CAD build for the part. Positions are in the model's coordinates, mm. A direction names the side the tool comes from. Give positions to 0.01 mm unless a question says otherwise; leave off trailing zeros. Loops run counter-clockwise (first coordinate to the right, second up) from the corner with the lowest first, then second, coordinate; pieces in that order, holes last.
Item 1: Drop flat-ended pins along their axis: P1, Ø1, axis at y = -1, z = 2, coming from the -X side; P2, Ø2, axis at y = -1.5, z = 1.5, coming from the -X side; P3, Ø1.5, axis at y = -0.5, z = 2, coming from the +X side. Give the stop position or say it passes through.
Item 2: Saw through at D-D on z = 0.25. Give the cut face in (x, y), plus the area to 3 significant figures.
Item 3: Saw through at C-C on x = 0. Give the cut face in (y, z), plus the area to 3 significant figures.
Item 4: Saw through at B-B on y = 0. Give the cut face in (x, z).
Item 5: Saw through at A-A on z = -2.25. Give the cut face in (x, y).
Item 6: Probe probe 1 along Y at (x, z) = (-1.2, 0.75); probe 2 along Y at (x, z) = (1.25, -0.25); probe 3 along Z at (x, y) = (0.6, -1.65). List the from-to ranges inside material, lowest first.
Item 7: Which spindle directions (+Z, -Z, +X, -X, +Y, -Y) get a long thin tool onto all of the face, cutting with end or side? Do faces 1 (the cylindrical face through (-1.5, 0.07, 2.28)), 2 (the flat face through (1.727, 0, 0.5)). Say none if no direction does.
from build123d import *

# Parameters (mm, degrees)
SKETCH1_R           = 2
BOSS_EXTRUDE1_DEPTH = 1
SKETCH2_R           = 1.5
BOSS_EXTRUDE2_DEPTH = 4
FILLET1_R           = 1.5
SKETCH3_W           = 0.5
SKETCH3_H           = 0.5
BOSS_EXTRUDE3_DEPTH = 4
FILLET2_R           = 0.2
FILLET3_R           = 0.1
FILLET4_R           = 0.1
CUT_EXTRUDE1_DEPTH  = 6


with BuildPart() as part:
    # Sketch1 → Boss-Extrude1 (new body)
    with BuildSketch(Plane.XY):
        Circle(SKETCH1_R)
    extrude(amount=BOSS_EXTRUDE1_DEPTH)

    # Sketch2 → Boss-Extrude2 (add)
    with BuildSketch(Plane.XY.offset(1)):
        Circle(SKETCH2_R)
    extrude(amount=BOSS_EXTRUDE2_DEPTH)

    # Fillet1
    fillet1_edges = [part.edges().sort_by_distance(p)[0] for p in [
        (-1.5, 0, 5),
    ]]
    fillet(fillet1_edges, radius=FILLET1_R)

    # Sketch3 → Boss-Extrude3 (add)
    with BuildSketch(Plane(origin=(0, 0, 0), x_dir=(-1, 0, 0), z_dir=(0, 0, -1))):
        with Locations((-1.27, 0)):
            Rectangle(SKETCH3_W, SKETCH3_H)
        with Locations((1.27, 0)):
            Rectangle(SKETCH3_W, SKETCH3_H)
    extrude(amount=BOSS_EXTRUDE3_DEPTH)

    # Fillet2
    fillet2_edges = [part.edges().sort_by_distance(p)[0] for p in [
        (-2, 0, 1),
    ]]
    fillet(fillet2_edges, radius=FILLET2_R)

    # Fillet3
    fillet3_edges = [part.edges().sort_by_distance(p)[0] for p in [
        (-1.5, 0, 1),
    ]]
    fillet(fillet3_edges, radius=FILLET3_R)

    # Fillet4
    fillet4_edges = [part.edges().sort_by_distance(p)[0] for p in [
        (1.02, -0.25, -2),
        (1.02, 0.25, -2),
        (1.52, 0.25, -2),
        (1.52, -0.25, -2),
        (-1.52, -0.25, -2),
        (-1.52, 0.25, -2),
        (-1.02, 0.25, -2),
        (-1.02, -0.25, -2),
    ]]
    fillet(fillet4_edges, radius=FILLET4_R)

    # Sketch5 → Cut-Extrude1 (cut, through all)
    with BuildSketch(Plane(origin=(0, 0, 0), x_dir=(-1, 0, 0), z_dir=(0, 0, -1))):
        with BuildLine():
            Line((-1.726643001, -1.009308647), (-1.726643001, 1.009308647))
            ThreePointArc((-1.726643001, 1.009308647), (-2, 0), (-1.726643001, -1.009308647))
        make_face()
    extrude(amount=-CUT_EXTRUDE1_DEPTH, mode=Mode.SUBTRACT)


solid = part.part
Results below:
1. P1: stops at x = -1.41
1. P2: stops at x = -1.85
1. P3: stops at x = 1.5
2. outline: (1.73, -1.01) - (1.73, 1.01) arc R2 ccw (long way) to start
2. area: 12.2 mm2
3. outline: (-2, 0) - (2, 0) - (2, 0.8) arc R0.2 ccw to (1.8, 1) - (1.6, 1) arc R0.1 cw to (1.5, 1.1) - (1.5, 3.5) arc R1.5 ccw to (-1.5, 3.5) - (-1.5, 1.1) arc R0.1 cw to (-1.6, 1) - (-1.8, 1) arc R0.2 ccw to (-2, 0.8) - close
3. area: 15.0 mm2
4. outline: (-2, 0) - (-1.52, 0) - (-1.52, -4) - (-1.02, -4) - (-1.02, 0) - (1.02, 0) - (1.02, -4) - (1.52, -4) - (1.52, 0) - (1.73, 0) - (1.73, 1) - (1.6, 1) arc R0.1 cw to (1.5, 1.1) - (1.5, 3.5) arc R1.5 ccw to (-1.5, 3.5) - (-1.5, 1.1) arc R0.1 cw to (-1.6, 1) - (-1.8, 1) arc R0.2 ccw to (-2, 0.8) - close
5. outline: (-1.52, -0.15) arc R0.1 ccw to (-1.42, -0.25) - (-1.12, -0.25) arc R0.1 ccw to (-1.02, -0.15) - (-1.02, 0.15) arc R0.1 ccw to (-1.12, 0.25) - (-1.42, 0.25) arc R0.1 ccw to (-1.52, 0.15) - close; (1.02, -0.15) arc R0.1 ccw to (1.12, -0.25) - (1.42, -0.25) arc R0.1 ccw to (1.52, -0.15) - (1.52, 0.15) arc R0.1 ccw to (1.42, 0.25) - (1.12, 0.25) arc R0.1 ccw to (1.02, 0.15) - close
6. probe 1: y = -1.6 to 1.6
6. probe 2: y = -0.25 to 0.25
6. probe 3: z = 0 to 1
7. face 1: +Z
7. face 2: +Z, -Z, +X, +Y, -Y
